Geometry: final body of the model. Coordinates: model frame, mm. Give positions to 0.01 mm unless a question says otherwise; leave off trailing zeros. Order: outer loops, then holes, each group sorted by start corner. A loop starts at its lowest first (then second) coordinate and runs counter-clockwise, first axis right, second up. Notation, with made-up numbers: (55.5, 59) -> (102.5, 59) arc R23 ccw to (102.5, 93) -> close; hole circle Ø4 at (48.25, 36). An arc over 180 degrees is marked (long way). Write item = value, one per line.
```python
from build123d import *

# Parameters (mm, degrees)
SKETCH_1_R           = 175
EXTRUDE_1_DEPTH      = 3
CUT_EXTRUDE_1_DEPTH  = 3
FILLET_1_R           = 5
FILLET_2_R           = 5
FILLET_3_R           = 5
SKETCH_5_R           = 1.5
CUT_EXTRUDE_4_DEPTH  = 3
SKETCH_10_R          = 12.5
SKETCH_10_R_2        = 1.3
CUT_EXTRUDE_13_DEPTH = 10
SKETCH_14_R          = 1.1
CUT_EXTRUDE_14_DEPTH = 10
SKETCH_12_R          = 1.5
CUT_EXTRUDE_17_DEPTH = 10
SKETCH_13_R          = 1.5
CUT_EXTRUDE_18_DEPTH = 5
SKETCH_17_R          = 1.1
CUT_EXTRUDE_19_DEPTH = 10
SKETCH_18_R          = 1.6
CUT_EXTRUDE_20_DEPTH = 10


with BuildPart() as part:
    # ｽｹｯﾁ1 → ﾎﾞｽ - 押し出し1 (new body)
    with BuildSketch(Plane.XY):
        Circle(SKETCH_1_R)
    extrude(amount=EXTRUDE_1_DEPTH)

    # ｽｹｯﾁ2 → ｶｯﾄ - 押し出し1 (cut)
    with BuildSketch(Plane.XY.offset(3)):
        with BuildLine():
            Line((-60, 115), (0, 115))
            Line((0, 115), (0, 175))
            ThreePointArc((0, 175), (-30.465194158, 172.327803749), (-60, 164.392822228))
            Line((-60, 164.392822228), (-60, 115))
        make_face()
        with BuildLine():
            Line((0, 175), (0, 115))
            Line((0, 115), (60, 115))
            Line((60, 115), (60, 164.392822228))
            ThreePointArc((60, 164.392822228), (30.465194158, 172.327803749), (0, 175))
        make_face()
        with BuildLine():
            Line((0, -175), (0, -115))
            Line((0, -115), (-60, -115))
            Line((-60, -115), (-60, -164.392822228))
            ThreePointArc((-60, -164.392822228), (-30.465194158, -172.327803749), (0, -175))
        make_face()
        with BuildLine():
            Line((60, -115), (0, -115))
            Line((0, -115), (0, -175))
            ThreePointArc((0, -175), (30.465194158, -172.327803749), (60, -164.392822228))
            Line((60, -164.392822228), (60, -115))
        make_face()
    extrude(amount=-CUT_EXTRUDE_1_DEPTH, mode=Mode.SUBTRACT)

    # ﾌｨﾚｯﾄ1
    fillet_1_edges = [part.edges().sort_by_distance(p)[0] for p in [
        (-60, 164.392822228, 1.5),
    ]]
    fillet(fillet_1_edges, radius=FILLET_1_R)

    # ﾌｨﾚｯﾄ2
    fillet_2_edges = [part.edges().sort_by_distance(p)[0] for p in [
        (-60, 115, 1.5),
        (60, 164.392822228, 1.5),
        (60, 115, 1.5),
    ]]
    fillet(fillet_2_edges, radius=FILLET_2_R)

    # ﾌｨﾚｯﾄ3
    fillet_3_edges = [part.edges().sort_by_distance(p)[0] for p in [
        (-60, -115, 1.5),
        (60, -115, 1.5),
        (60, -164.392822228, 1.5),
        (-60, -164.392822228, 1.5),
    ]]
    fillet(fillet_3_edges, radius=FILLET_3_R)

    # ｽｹｯﾁ5 → ｶｯﾄ - 押し出し4 (cut)
    with BuildSketch(Plane.XY.offset(3)):
        with Locations((-100, -115)):
            Circle(SKETCH_5_R)
        with Locations((100, -115)):
            Circle(SKETCH_5_R)
        with Locations((100, 115)):
            Circle(SKETCH_5_R)
        with Locations((-100, 115)):
            Circle(SKETCH_5_R)
    extrude(amount=-CUT_EXTRUDE_4_DEPTH, mode=Mode.SUBTRACT)

    # ｽｹｯﾁ10 → ｶｯﾄ - 押し出し13 (cut)
    with BuildSketch(Plane.XY.offset(3)):
        with Locations((-150, 0)):
            Circle(SKETCH_10_R)
        with Locations((150, 0)):
            Circle(SKETCH_10_R)
        Circle(SKETCH_10_R)
        with Locations((132.5, 0)):
            Circle(SKETCH_10_R_2)
        with Locations((158.75, 15.155444566)):
            Circle(SKETCH_10_R_2)
        with Locations((158.75, -15.155444566)):
            Circle(SKETCH_10_R_2)
        with Locations((-15.155444566, 8.75)):
            Circle(SKETCH_10_R_2)
        with Locations((15.155444566, 8.75)):
            Circle(SKETCH_10_R_2)
        with Locations((0, -17.5)):
            Circle(SKETCH_10_R_2)
        with Locations((-158.75, 15.155444566)):
            Circle(SKETCH_10_R_2)
        with Locations((-158.75, -15.155444566)):
            Circle(SKETCH_10_R_2)
        with Locations((-132.632898389, 0)):
            Circle(SKETCH_10_R_2)
    extrude(amount=-CUT_EXTRUDE_13_DEPTH, mode=Mode.SUBTRACT)

    # ｽｹｯﾁ14 → ｶｯﾄ - 押し出し14 (cut)
    with BuildSketch(Plane.XY.offset(3)):
        with Locations((-170, 5)):
            Circle(SKETCH_14_R)
        with Locations((-170, -5)):
            Circle(SKETCH_14_R)
        with Locations((-114.933514447, 125.360628815)):
            Circle(SKETCH_14_R)
        with Locations((-122.102620524, 118.388977786)):
            Circle(SKETCH_14_R)
        with Locations((-122.102620524, -118.388977786)):
            Circle(SKETCH_14_R)
        with Locations((-114.933514447, -125.360628815)):
            Circle(SKETCH_14_R)
    extrude(amount=-CUT_EXTRUDE_14_DEPTH, mode=Mode.SUBTRACT)

    # ｽｹｯﾁ12 → ｶｯﾄ - 押し出し17 (cut)
    with BuildSketch(Plane.XY.offset(3)):
        with Locations((-15, 94)):
            Circle(SKETCH_12_R)
        with Locations((15, 94)):
            Circle(SKETCH_12_R)
        with Locations((-15, -94)):
            Circle(SKETCH_12_R)
        with Locations((15, -94)):
            Circle(SKETCH_12_R)
    extrude(amount=-CUT_EXTRUDE_17_DEPTH, mode=Mode.SUBTRACT)

    # ｽｹｯﾁ13 → ｶｯﾄ - 押し出し18 (cut)
    with BuildSketch(Plane.XY.offset(3)):
        with Locations((-28, -104)):
            Circle(SKETCH_13_R)
        with Locations((-46, -104)):
            Circle(SKETCH_13_R)
        with Locations((-46, 104)):
            Circle(SKETCH_13_R)
        with Locations((-28, 104)):
            Circle(SKETCH_13_R)
    extrude(amount=-CUT_EXTRUDE_18_DEPTH, mode=Mode.SUBTRACT)

    # ｽｹｯﾁ17 → ｶｯﾄ - 押し出し19 (cut)
    with BuildSketch(Plane.XY.offset(3)):
        with Locations((170, 5)):
            Circle(SKETCH_17_R)
        with Locations((170, -5)):
            Circle(SKETCH_17_R)
        with Locations((114.933514447, 125.360628815)):
            Circle(SKETCH_17_R)
        with Locations((122.102620524, 118.388977786)):
            Circle(SKETCH_17_R)
        with Locations((122.102620524, -118.388977786)):
            Circle(SKETCH_17_R)
        with Locations((114.933514447, -125.360628815)):
            Circle(SKETCH_17_R)
    extrude(amount=-CUT_EXTRUDE_19_DEPTH, mode=Mode.SUBTRACT)

    # ｽｹｯﾁ18 → ｶｯﾄ - 押し出し20 (cut)
    with BuildSketch(Plane.XY.offset(3)):
        with Locations((-50, 38.25)):
            Circle(SKETCH_18_R)
        with Locations((-80.5, 38.25)):
            Circle(SKETCH_18_R)
        with Locations((-50, -38.25)):
            Circle(SKETCH_18_R)
    extrude(amount=-CUT_EXTRUDE_20_DEPTH, mode=Mode.SUBTRACT)


solid = part.part
```
1) First-contact query: P1, Ø3.5, axis at x = 132.5, y = 0, coming from the +Z side; P2, Ø20, axis at x = 150, y = 0, coming from the -Z side; P3, Ø1, axis at x = -122.5, z = 2, coming from the -Y side; P4, Ø1.5, axis at x = -10, z = 1, coming from the -Y side. Flat tips, straight axial feed; report the tip coordinate or a pass-through.
Check sheet entries:
P1 = 3
P2 = through
P3 = -125.46
P4 = -115
2) Section query B-B (z = 1.9). Count the separate pieces of the cut face and the enclosed holes in it, plus the area to 3 significant figures.
Check sheet entries:
separate_pieces = 1
enclosed_holes = 39
area = 80,900 mm²
3) Mould query, pull axis X, two halves, no side actions, for faces 1 (the face through (-174.976, 2.887, 1.479)), 2 (the face through (-2, -34, 3)), 3 (the face through (11.923, 3.755, 1.521)), 4 (the face through (-138.077, 3.755, 1.521)). Classes: +X half, -X half, draft (parallel to the pull), parting line (faces both ways), or undercut.
Check sheet entries:
face_1 = -X half
face_2 = draft
face_3 = undercut
face_4 = undercut
4) Section query A-A (x = 150). Output: boundary loops of the cut face in (y, z).
Check sheet entries:
outline = (-90.14, 0) -> (-12.5, 0) -> (-12.5, 3) -> (-90.14, 3) -> close; (12.5, 0) -> (90.14, 0) -> (90.14, 3) -> (12.5, 3) -> close
5) Line query: line 1 (Y direction, x = -46, z = 2.25); line 2 (Y direction, x = -148.5, z = 1.75); line 3 (Y direction, x = 17, z = 0.45). Output: solid intervals per line, ascending. Write a range as from..to.
Check sheet entries:
line_1 = -115..-105.5, -102.5..102.5, 105.5..115
line_2 = -92.59..-12.41, 12.41..92.59
line_3 = -115..115
6) Section query D-D (y = 83). Output: boundary loops of the cut face in (x, z), plus the area to 3 significant figures.
Check sheet entries:
outline = (-154.06, 0) -> (154.06, 0) -> (154.06, 3) -> (-154.06, 3) -> close
area = 924 mm²
7) Section query C-C (x = 34). Output: boundary loops of the cut face in (y, z).
Check sheet entries:
outline = (-115, 0) -> (115, 0) -> (115, 3) -> (-115, 3) -> close
